from build123d import *

# Parameters (mm, degrees)
F2_W     = 3.25
F2_H     = 3.25
F3_DEPTH = 30.001


with BuildPart() as f1:
    # F0 (on Front) → F1 (revolve)
    with BuildSketch(Plane.XZ):
        with BuildLine():
            Line((0, 30), (0, 0))
            Line((0, 0), (12.5, 0))
            add(Edge.make_bspline(
                [(12.5, 30), (9.055907, 25.34046), (6.907983, 14.663109), (9.128126, 5.333321), (12.5, 0)],
                knots=[0, 0, 0, 0, 15.66046, 31.32092, 31.32092, 31.32092, 31.32092], degree=3))
            Line((12.5, 30), (0, 30))
        make_face()
    revolve(axis=Axis((0, 0, 15), (0, 0, 1)))

    # F2 (on face) → F3 (cut, through all)
    with BuildSketch(Plane.XY.offset(30)):
        Rectangle(F2_W, F2_H)
    extrude(amount=-F3_DEPTH, mode=Mode.SUBTRACT)


solid = f1.part
Can you work these out from the model? Positions are in its coordinate system, mm. A direction names the side the tool comes from. Give positions to 0.01 mm unless a question says otherwise; leave off trailing zeros. Return JSON: item names as keys, results as strings.
Q1. I need wall thicknesses on probe 1 along Y at (x, z) = (-1, 28.5) (3 decimals); probe 2 along X at (y, z) = (1, 3) (3 decimals); probe 3 along X at (y, z) = (-0.5, 27.5) (3 decimals). Which ranges of each line are inside material? Lowest first, please.
Checks:
{"probe 1": "y = -11.442 to -1.625, 1.625 to 11.442", "probe 2": "x = -10.756 to -1.625, 1.625 to 10.756", "probe 3": "x = -10.893 to -1.625, 1.625 to 10.893"}
Q2. On a 3-axis mill with a long thin cutter (end or side, diameter ignored), from which of +Z, -Z, +X, -X, +Y, -Y can I reach the whole of each face in a straight line? I mean faces 4 (the face through (0, -3, 0)), 5 (the face through (0, -1.625, 15)). Say none if no direction works.
Checks:
{"face 4": "-Z, +X, -X, +Y, -Y", "face 5": "+Z, -Z"}
Q3. For pin 1 Ø3.5 at (x, z) = (-0.5, 16) entering from +Y; pin 2 Ø5 at (x, z) = (-6.5, 22) entering from +Y; pin 3 Ø5 at (x, z) = (5, 5.5) entering from -Y, each with a flat end and sliding along its axis, tell me the tip position at first contact or that it passes through.
Checks:
{"pin 1": "stops at y = 8.1", "pin 2": "stops at y = 8.04", "pin 3": "stops at y = -9.96"}
Q4. We'd pull the mould along X, two halves only. Please class faces 1 (the face through (0, 1.625, 15)), 2 (the face through (1.625, 0, 15)), 3 (the face through (0, -3, 30)): released by +X, released by -X, zero draft, split by the parting line, or undercut.
Checks:
{"face 1": "undercut", "face 2": "undercut", "face 3": "zero draft"}
